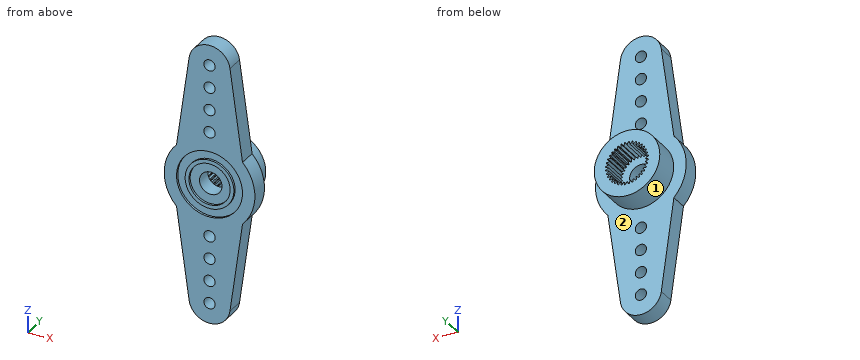
```python
from build123d import *

# Parameters (mm, degrees)
BOSS_EXTRUDE1_DEPTH                                = 2.35
SKETCH2_R                                          = 4.375
BOSS_EXTRUDE2_DEPTH                                = 3.4
CUT_EXTRUDE1_DEPTH                                 = 3.4
F_8_8_8_8_DIAMETER_HOLE1_D                         = 8.8
F_8_8_8_8_DIAMETER_HOLE1_DEPTH                     = 0.3
SKETCH6_W                                          = 3.25
SKETCH6_H                                          = 0.3
F_1_5_1_5_DIAMETER_HOLE1_D                         = 1.5
F_1_5_1_5_DIAMETER_HOLE1_DEPTH                     = 2.35
CBORE_FOR_M2_5_HEX_HEAD_MACHINE_SCREW1_D           = 3
CBORE_FOR_M2_5_HEX_HEAD_MACHINE_SCREW1_DEPTH       = 5.75
CBORE_FOR_M2_5_HEX_HEAD_MACHINE_SCREW1_CBORE_D     = 5.5
CBORE_FOR_M2_5_HEX_HEAD_MACHINE_SCREW1_CBORE_DEPTH = 0.3


with BuildPart() as part:
    # Sketch1 → Boss-Extrude1 (new body)
    with BuildSketch(Plane(origin=(0, 2.35, 0), x_dir=(1, 0, 0), z_dir=(0, 1, 0))):
        with BuildLine():
            Line((2.724307673, -16.32503027), (4.4, -4.152408939))
            ThreePointArc((4.4, -4.152408939), (6.05, 0), (4.4, 4.152408939))
            Line((4.4, 4.152408939), (2.724307673, 16.32503027))
            ThreePointArc((2.724307673, 16.32503027), (0, 18.7), (-2.724307673, 16.32503027))
            Line((-2.724307673, 16.32503027), (-4.4, 4.152408939))
            ThreePointArc((-4.4, 4.152408939), (-6.05, 0), (-4.4, -4.152408939))
            Line((-4.4, -4.152408939), (-2.724307673, -16.32503027))
            ThreePointArc((-2.724307673, -16.32503027), (0, -18.7), (2.724307673, -16.32503027))
        make_face()
    extrude(amount=-BOSS_EXTRUDE1_DEPTH)

    # Sketch2 → Boss-Extrude2 (add)
    with BuildSketch(Plane(origin=(0, 2.35, 0), x_dir=(-1, 0, 0), z_dir=(0, 1, 0))):
        Circle(SKETCH2_R)
    extrude(amount=BOSS_EXTRUDE2_DEPTH)

    # Sketch3 → Cut-Extrude1 (cut)
    with BuildSketch(Plane(origin=(0, 5.75, 0), x_dir=(-1, 0, 0), z_dir=(0, 1, 0))):
        with BuildLine():
            Line((0.687336745, 2.765875666), (0.425438035, 2.412778995))
            Line((0.425438035, 2.412778995), (0.300099924, 2.834155965))
            ThreePointArc((0.300099924, 2.834155965), (0.248393867, 2.83915489), (0.196605286, 2.843210573))
            Line((0.196605286, 2.843210573), (0, 2.45))
            Line((0, 2.45), (-0.196605286, 2.843210573))
            ThreePointArc((-0.196605286, 2.843210573), (-0.248393867, 2.83915489), (-0.300099924, 2.834155965))
            Line((-0.300099924, 2.834155965), (-0.425438035, 2.412778995))
            Line((-0.425438035, 2.412778995), (-0.687336745, 2.765875666))
            ThreePointArc((-0.687336745, 2.765875666), (-0.737634279, 2.752888605), (-0.787686751, 2.738986963))
            Line((-0.787686751, 2.738986963), (-0.837949351, 2.302246921))
            Line((-0.837949351, 2.302246921), (-1.157183824, 2.604501026))
            ThreePointArc((-1.157183824, 2.604501026), (-1.204462046, 2.582977193), (-1.251340114, 2.560595228))
            Line((-1.251340114, 2.560595228), (-1.225, 2.121762239))
            Line((-1.225, 2.121762239), (-1.591870459, 2.363989941))
            ThreePointArc((-1.591870459, 2.363989941), (-1.634692844, 2.334583326), (-1.676972141, 2.304401102))
            Line((-1.676972141, 2.304401102), (-1.574829644, 1.876808886))
            Line((-1.574829644, 1.876808886), (-1.978188915, 2.051650218))
            ThreePointArc((-1.978188915, 2.051650218), (-2.015254326, 2.015254326), (-2.051650218, 1.978188915))
            Line((-2.051650218, 1.978188915), (-1.876808886, 1.574829644))
            Line((-1.876808886, 1.574829644), (-2.304401102, 1.676972141))
            ThreePointArc((-2.304401102, 1.676972141), (-2.334583326, 1.634692844), (-2.363989941, 1.591870459))
            Line((-2.363989941, 1.591870459), (-2.121762239, 1.225))
            Line((-2.121762239, 1.225), (-2.560595228, 1.251340114))
            ThreePointArc((-2.560595228, 1.251340114), (-2.582977193, 1.204462046), (-2.604501026, 1.157183824))
            Line((-2.604501026, 1.157183824), (-2.302246921, 0.837949351))
            Line((-2.302246921, 0.837949351), (-2.738986963, 0.787686751))
            ThreePointArc((-2.738986963, 0.787686751), (-2.752888605, 0.737634279), (-2.765875666, 0.687336745))
            Line((-2.765875666, 0.687336745), (-2.412778995, 0.425438035))
            Line((-2.412778995, 0.425438035), (-2.834155965, 0.300099924))
            ThreePointArc((-2.834155965, 0.300099924), (-2.83915489, 0.248393867), (-2.843210573, 0.196605286))
            Line((-2.843210573, 0.196605286), (-2.45, 0))
            Line((-2.45, 0), (-2.843210573, -0.196605286))
            ThreePointArc((-2.843210573, -0.196605286), (-2.83915489, -0.248393867), (-2.834155965, -0.300099924))
            Line((-2.834155965, -0.300099924), (-2.412778995, -0.425438035))
            Line((-2.412778995, -0.425438035), (-2.765875666, -0.687336745))
            ThreePointArc((-2.765875666, -0.687336745), (-2.752888605, -0.737634279), (-2.738986963, -0.787686751))
            Line((-2.738986963, -0.787686751), (-2.302246921, -0.837949351))
            Line((-2.302246921, -0.837949351), (-2.604501026, -1.157183824))
            ThreePointArc((-2.604501026, -1.157183824), (-2.582977193, -1.204462046), (-2.560595228, -1.251340114))
            Line((-2.560595228, -1.251340114), (-2.121762239, -1.225))
            Line((-2.121762239, -1.225), (-2.363989941, -1.591870459))
            ThreePointArc((-2.363989941, -1.591870459), (-2.334583326, -1.634692844), (-2.304401102, -1.676972141))
            Line((-2.304401102, -1.676972141), (-1.876808886, -1.574829644))
            Line((-1.876808886, -1.574829644), (-2.051650218, -1.978188915))
            ThreePointArc((-2.051650218, -1.978188915), (-2.015254326, -2.015254326), (-1.978188915, -2.051650218))
            Line((-1.978188915, -2.051650218), (-1.574829644, -1.876808886))
            Line((-1.574829644, -1.876808886), (-1.676972141, -2.304401102))
            ThreePointArc((-1.676972141, -2.304401102), (-1.634692844, -2.334583326), (-1.591870459, -2.363989941))
            Line((-1.591870459, -2.363989941), (-1.225, -2.121762239))
            Line((-1.225, -2.121762239), (-1.251340114, -2.560595228))
            ThreePointArc((-1.251340114, -2.560595228), (-1.204462046, -2.582977193), (-1.157183824, -2.604501026))
            Line((-1.157183824, -2.604501026), (-0.837949351, -2.302246921))
            Line((-0.837949351, -2.302246921), (-0.787686751, -2.738986963))
            ThreePointArc((-0.787686751, -2.738986963), (-0.737634279, -2.752888605), (-0.687336745, -2.765875666))
            Line((-0.687336745, -2.765875666), (-0.425438035, -2.412778995))
            Line((-0.425438035, -2.412778995), (-0.300099924, -2.834155965))
            ThreePointArc((-0.300099924, -2.834155965), (-0.248393867, -2.83915489), (-0.196605286, -2.843210573))
            Line((-0.196605286, -2.843210573), (0, -2.45))
            Line((0, -2.45), (0.196605286, -2.843210573))
            ThreePointArc((0.196605286, -2.843210573), (0.248393867, -2.83915489), (0.300099924, -2.834155965))
            Line((0.300099924, -2.834155965), (0.425438035, -2.412778995))
            Line((0.425438035, -2.412778995), (0.687336745, -2.765875666))
            ThreePointArc((0.687336745, -2.765875666), (0.737634279, -2.752888605), (0.787686751, -2.738986963))
            Line((0.787686751, -2.738986963), (0.837949351, -2.302246921))
            Line((0.837949351, -2.302246921), (1.157183824, -2.604501026))
            ThreePointArc((1.157183824, -2.604501026), (1.204462046, -2.582977193), (1.251340114, -2.560595228))
            Line((1.251340114, -2.560595228), (1.225, -2.121762239))
            Line((1.225, -2.121762239), (1.591870459, -2.363989941))
            ThreePointArc((1.591870459, -2.363989941), (1.634692844, -2.334583326), (1.676972141, -2.304401102))
            Line((1.676972141, -2.304401102), (1.574829644, -1.876808886))
            Line((1.574829644, -1.876808886), (1.978188915, -2.051650218))
            ThreePointArc((1.978188915, -2.051650218), (2.015254326, -2.015254326), (2.051650218, -1.978188915))
            Line((2.051650218, -1.978188915), (1.876808886, -1.574829644))
            Line((1.876808886, -1.574829644), (2.304401102, -1.676972141))
            ThreePointArc((2.304401102, -1.676972141), (2.334583326, -1.634692844), (2.363989941, -1.591870459))
            Line((2.363989941, -1.591870459), (2.121762239, -1.225))
            Line((2.121762239, -1.225), (2.560595228, -1.251340114))
            ThreePointArc((2.560595228, -1.251340114), (2.582977193, -1.204462046), (2.604501026, -1.157183824))
            Line((2.604501026, -1.157183824), (2.302246921, -0.837949351))
            Line((2.302246921, -0.837949351), (2.738986963, -0.787686751))
            ThreePointArc((2.738986963, -0.787686751), (2.752888605, -0.737634279), (2.765875666, -0.687336745))
            Line((2.765875666, -0.687336745), (2.412778995, -0.425438035))
            Line((2.412778995, -0.425438035), (2.834155965, -0.300099924))
            ThreePointArc((2.834155965, -0.300099924), (2.83915489, -0.248393867), (2.843210573, -0.196605286))
            Line((2.843210573, -0.196605286), (2.45, 0))
            Line((2.45, 0), (2.843210573, 0.196605286))
            ThreePointArc((2.843210573, 0.196605286), (2.83915489, 0.248393867), (2.834155965, 0.300099924))
            Line((2.834155965, 0.300099924), (2.412778995, 0.425438035))
            Line((2.412778995, 0.425438035), (2.765875666, 0.687336745))
            ThreePointArc((2.765875666, 0.687336745), (2.752888605, 0.737634279), (2.738986963, 0.787686751))
            Line((2.738986963, 0.787686751), (2.302246921, 0.837949351))
            Line((2.302246921, 0.837949351), (2.604501026, 1.157183824))
            ThreePointArc((2.604501026, 1.157183824), (2.582977193, 1.204462046), (2.560595228, 1.251340114))
            Line((2.560595228, 1.251340114), (2.121762239, 1.225))
            Line((2.121762239, 1.225), (2.363989941, 1.591870459))
            ThreePointArc((2.363989941, 1.591870459), (2.334583326, 1.634692844), (2.304401102, 1.676972141))
            Line((2.304401102, 1.676972141), (1.876808886, 1.574829644))
            Line((1.876808886, 1.574829644), (2.051650218, 1.978188915))
            ThreePointArc((2.051650218, 1.978188915), (2.015254326, 2.015254326), (1.978188915, 2.051650218))
            Line((1.978188915, 2.051650218), (1.574829644, 1.876808886))
            Line((1.574829644, 1.876808886), (1.676972141, 2.304401102))
            ThreePointArc((1.676972141, 2.304401102), (1.634692844, 2.334583326), (1.591870459, 2.363989941))
            Line((1.591870459, 2.363989941), (1.225, 2.121762239))
            Line((1.225, 2.121762239), (1.251340114, 2.560595228))
            ThreePointArc((1.251340114, 2.560595228), (1.204462046, 2.582977193), (1.157183824, 2.604501026))
            Line((1.157183824, 2.604501026), (0.837949351, 2.302246921))
            Line((0.837949351, 2.302246921), (0.787686751, 2.738986963))
            ThreePointArc((0.787686751, 2.738986963), (0.737634279, 2.752888605), (0.687336745, 2.765875666))
        make_face()
    extrude(amount=-CUT_EXTRUDE1_DEPTH, mode=Mode.SUBTRACT)

    # Ø8.8 (8.8) Diameter Hole1
    with Locations(Plane(origin=(0, 0, 0), x_dir=(-1, 0, 0), z_dir=(0, -1, 0))):
        with Locations((0, 0)):
            Hole(F_8_8_8_8_DIAMETER_HOLE1_D / 2, depth=F_8_8_8_8_DIAMETER_HOLE1_DEPTH)

    # Sketch6 → Revolve1 (revolve)
    with BuildSketch(Plane.XY):
        with Locations((1.625, 0.15)):
            Rectangle(SKETCH6_W, SKETCH6_H)
    revolve(axis=Axis((0, 0.3, 0), (0, -1, 0)))

    # Ø1.5 (1.5) Diameter Hole1
    with Locations(Plane(origin=(0, 2.35, 0), x_dir=(1, 0, 0), z_dir=(0, 1, 0))):
        with Locations((0, -7), (0, 16), (0, -10), (0, -13), (0, -16), (0, 13), (0, 10), (0, 7)):
            Hole(F_1_5_1_5_DIAMETER_HOLE1_D / 2, depth=F_1_5_1_5_DIAMETER_HOLE1_DEPTH)

    # CBORE for M2.5 Hex Head Machine Screw1
    with Locations(Plane(origin=(0, 0, 0), x_dir=(-1, 0, 0), z_dir=(0, -1, 0))):
        with Locations((0, 0)):
            CounterBoreHole(CBORE_FOR_M2_5_HEX_HEAD_MACHINE_SCREW1_D / 2, CBORE_FOR_M2_5_HEX_HEAD_MACHINE_SCREW1_CBORE_D / 2, CBORE_FOR_M2_5_HEX_HEAD_MACHINE_SCREW1_CBORE_DEPTH, depth=CBORE_FOR_M2_5_HEX_HEAD_MACHINE_SCREW1_DEPTH)


solid = part.part
```
Model file for the job. Use its own axes, mm. Face numbers are marked on the shaded views. Coordinates: 2 decimals unless noted, no trailing zeros. Order: outer loops, then holes, each group sorted by start corner. A loop starts at its lowest first (then second) coordinate and runs counter-clockwise, first axis right, second up. Notation, with made-up numbers: (20.5, 41) -> (76.5, 41) arc R10 ccw to (76.5, 58) -> close; hole circle Ø7 at (83, 19.25). An arc over 180 degrees is marked (long way). Answer as a JSON object with one key per item and string values. Group by question number.
1) Cut at D-D, the plane x = 5.25. Write the cut outline in (y, z).
2) Drill centre lines: L1, parallel to Y at x = 2.5, z = -6; L2, parallel to X at y = 3.95, z = -2; L3, parallel to Y at x = 0.25, z = 4. Where is each one in solid material? Low to high.
3) Pull direction Z, two halves, no side cores. Call the marked faces 1 and 2: +Z half, -Z half, draft (parallel to the pull), parting line (faces both ways), or undercut.
4) Flat gauge pins, fed straight in: pin 1 (1.4 mm diameter, centred on x = 0, z = -13, fed in from -Y); pin 2 (4 mm diameter, centred on x = -0.5, z = -11.5, fed in from +Y); pin 3 (3.5 mm diameter, centred on x = 0, z = 0, fed in from -Y). Where does each tip first touch, or does it go through?
5) Cut at A-A, the plane y = 1.8. Count the separate pieces of the cut face and the enclosed holes in it, then the cut area to 3 significant figures.
6) Cut at C-C, the plane z = -16. Write the cut outline in (x, y).
7) Cut at B-B, the plane z = -10. Write the cut outline in (x, y).
Check values:
{
 "1": {"outline": "(0, -3.01) -> (2.35, -3.01) -> (2.35, 3.01) -> (0, 3.01) -> close"},
 "2": {"L1": "y = 0 to 2.35", "L2": "x = -3.89 to -2.03, -1.86 to -1.6, 1.6 to 1.86, 2.03 to 3.89", "L3": "y = 0.3 to 5.75"},
 "3": {"face 1": "parting line", "face 2": "draft"},
 "4": {"pin 1": "passes through", "pin 2": "stops at y = 2.35", "pin 3": "stops at y = 0.3"},
 "5": {"separate pieces": "1", "enclosed holes": "9", "area": "264 mm²"},
 "6": {"outline": "(-2.77, 0) -> (-0.75, 0) -> (-0.75, 2.35) -> (-2.77, 2.35) -> close; (0.75, 0) -> (2.77, 0) -> (2.77, 2.35) -> (0.75, 2.35) -> close"},
 "7": {"outline": "(-3.6, 0) -> (-0.75, 0) -> (-0.75, 2.35) -> (-3.6, 2.35) -> close; (0.75, 0) -> (3.6, 0) -> (3.6, 2.35) -> (0.75, 2.35) -> close"}
}
